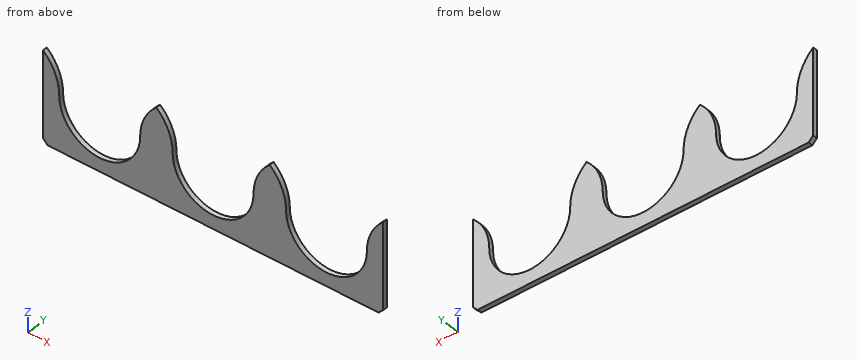
from build123d import *

# Parameters (mm, degrees)
BOSS_EXTRUDE1_DEPTH = 6.35


with BuildPart() as part:
    # Sketch1 → Boss-Extrude1 (new body)
    with BuildSketch(Plane(origin=(0, 0, 0), x_dir=(1, 0, 0), z_dir=(0, 1, 0))):
        with BuildLine():
            ThreePointArc((13.694028754, -34.373994235), (19.562343483, -61.559675463), (36.122228754, -83.903994235))
            Line((36.122228754, -83.903994235), (36.122228754, 39.921005765))
            Line((36.122228754, 39.921005765), (-114.144171246, 39.921005765))
            Line((-114.144171246, 39.921005765), (-120.494171246, 33.571005765))
            Line((-120.494171246, 33.571005765), (-120.494171246, -83.903994235))
            ThreePointArc((-120.494171246, -83.903994235), (-103.934285976, -61.559675463), (-98.065971246, -34.373994235))
            ThreePointArc((-98.065971246, -34.373994235), (-42.185971246, 21.506005765), (13.694028754, -34.373994235))
        make_face()
        with BuildLine():
            Line((36.122228754, 39.921005765), (36.122228754, -83.903994235))
            ThreePointArc((36.122228754, -83.903994235), (52.682114024, -61.559675463), (58.550428754, -34.373994235))
            ThreePointArc((58.550428754, -34.373994235), (114.430428754, 21.506005765), (170.310428754, -34.373994235))
            ThreePointArc((170.310428754, -34.373994235), (176.178743483, -61.559675463), (192.738628754, -83.903994235))
            Line((192.738628754, -83.903994235), (192.738628754, 39.921005765))
            Line((192.738628754, 39.921005765), (36.122228754, 39.921005765))
        make_face()
        with BuildLine():
            Line((343.055828754, 39.921005765), (192.738628754, 39.921005765))
            Line((192.738628754, 39.921005765), (192.738628754, -83.903994235))
            ThreePointArc((192.738628754, -83.903994235), (209.316728258, -61.564916677), (215.192228754, -34.373994235))
            ThreePointArc((215.192228754, -34.373994235), (271.072228754, 21.506005765), (326.952228754, -34.373994235))
            ThreePointArc((326.952228754, -34.373994235), (332.827729249, -61.564916677), (349.405828754, -83.903994235))
            Line((349.405828754, -83.903994235), (349.405828754, 33.571005765))
            Line((349.405828754, 33.571005765), (343.055828754, 39.921005765))
        make_face()
    extrude(amount=-BOSS_EXTRUDE1_DEPTH)


solid = part.part
Here's how the part is built. I have some questions about the finished solid (model axes, mm). Coordinates: 2 decimals unless noted, no trailing zeros. Write each loop counter-clockwise with the first axis right and the second up, starting at its lowest first coordinate (ties: lowest second). Pieces come first, ordered by that corner, then holes.
Item 1: I want a section at A-A on y = -1.5. Write out the boundary of the cut face in (x, z).
Item 2: I want a section at B-B on z = 13.5. Write out the boundary of the cut face in (x, y).
Item 3: I want a section at C-C on z = 42. Write out the boundary of the cut face in (x, y).
Item 4: If I drill on line 1 (X direction, y = -6, z = -2); line 2 (X direction, y = -4.5, z = 34.5); line 3 (Z direction, x = -43.5, y = -0.75), over which ranges is the centre line in solid material (lowest first)?
Item 5: I want a section at D-D on x = 293. Write out the boundary of the cut face in (y, z), and give its area (3 significant figures).
Findings below:
1. outline: (-120.49, -33.57) - (-114.14, -39.92) - (343.06, -39.92) - (349.41, -33.57) - (349.41, 83.9) arc R65.86 ccw to (326.95, 34.37) arc R55.88 cw to (215.19, 34.37) arc R65.86 ccw to (192.74, 83.9) arc R65.9 ccw to (170.31, 34.37) arc R55.88 cw to (58.55, 34.37) arc R65.9 ccw to (36.12, 83.9) arc R65.9 ccw to (13.69, 34.37) arc R55.88 cw to (-98.07, 34.37) arc R65.9 ccw to (-120.49, 83.9) - close
2. outline: (-120.49, -6.35) - (-94.02, -6.35) - (-94.02, 0) - (-120.49, 0) - close; (9.65, -6.35) - (62.6, -6.35) - (62.6, 0) - (9.65, 0) - close; (166.27, -6.35) - (219.24, -6.35) - (219.24, 0) - (166.27, 0) - close; (322.91, -6.35) - (349.41, -6.35) - (349.41, 0) - (322.91, 0) - close
3. outline: (-120.49, -6.35) - (-98.51, -6.35) - (-98.51, 0) - (-120.49, 0) - close; (14.14, -6.35) - (58.11, -6.35) - (58.11, 0) - (14.14, 0) - close; (170.75, -6.35) - (214.75, -6.35) - (214.75, 0) - (170.75, 0) - close; (327.4, -6.35) - (349.41, -6.35) - (349.41, 0) - (327.4, 0) - close
4. line 1: x = -120.49 to -84.61, 0.23 to 72.01, 156.85 to 228.65, 313.49 to 349.41
4. line 2: x = -120.49 to -98.07, 13.69 to 58.55, 170.31 to 215.19, 326.95 to 349.41
4. line 3: z = -39.92 to -21.49
5. outline: (-6.35, -39.92) - (0, -39.92) - (0, -17.02) - (-6.35, -17.02) - close
5. area: 145 mm2
